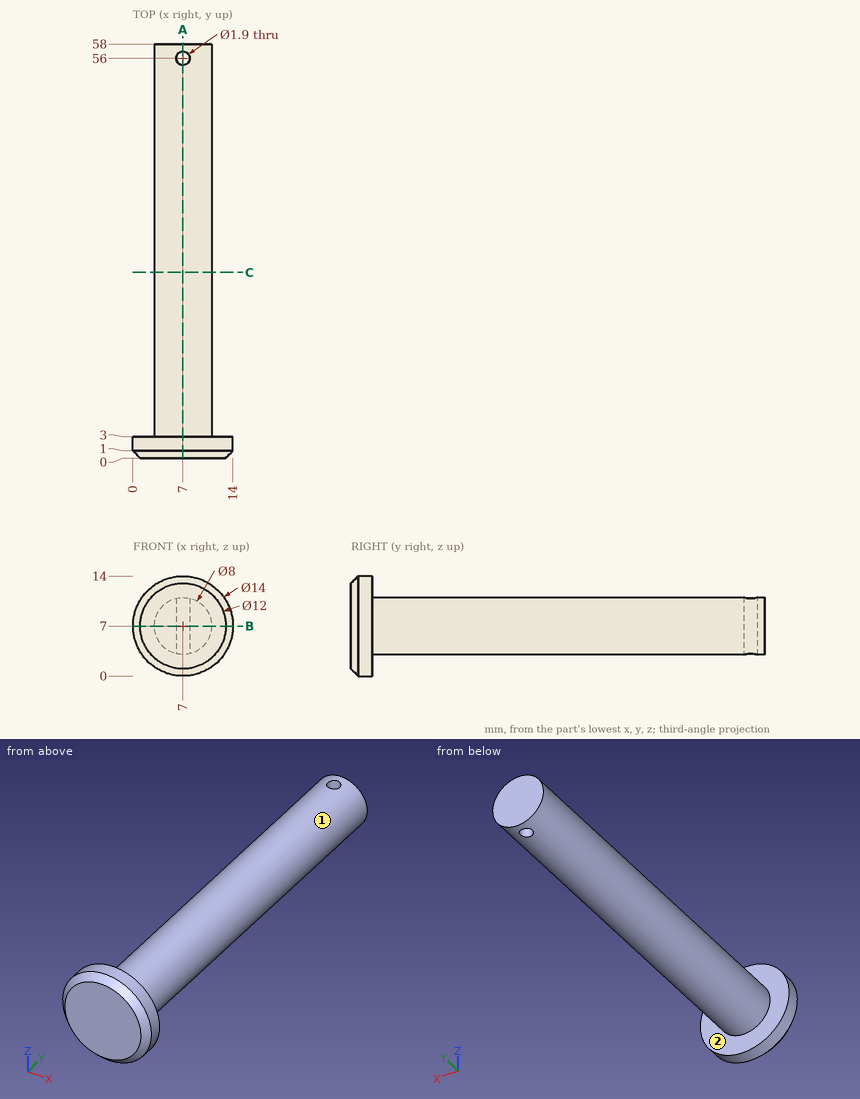
Answer from the drawing. Dimensions are ordinates in mm from the lowest x, y and z of the part. Coordinates: 2 decimals unless noted, no trailing zeros. Order: outer loops, then holes, each group sorted by start corner. A loop starts at its lowest first (then second) coordinate and runs counter-clockwise, first axis right, second up. Notation, with made-up numbers: M 41,4 L 70,4 A30 ccw 70,28 Z; hole C 27,69.5 d11. An arc over 180 degrees is marked long. Put each result on its own line as item: value. Start each with the question number.
Item 1: The mould has two halves that part along Z. Classify the marked faces 1 and 2: +Z half, -Z half, draft (parallel to the pull), parting line (faces both ways), or undercut.
Item 2: Section C-C, the plane y = 26 is taken. Determine the outline of the cut face in (x, z), plus the area to 3 significant figures.
Item 3: Given pin 1 Ø5 at (x, y) = (8, 21.5) entering from -Z; pin 2 Ø1.5 at (y, z) = (9, 7.5) entering from +X; pin 3 Ø6 at (x, y) = (8.5, 18) entering from +Z, each flat-ended and moving along its own axis, determine where each tip first touches the part or whether it passes through.
Item 4: Consider probe 1 along Y at (x, z) = (7, 5.75); probe 2 along Y at (x, z) = (11, 8.75); probe 3 along Z at (x, y) = (7.25, 49). Determine where each line is inside the solid, lowest interval first. Write a range as [from, to].
Item 5: Section A-A, the plane x = 7 is taken. Determine the outline of the cut face in (y, z).
Item 6: Section B-B, the plane z = 7 is taken. Determine the outline of the cut face in (x, y).
Computed:
1. face 1: parting line
1. face 2: draft
2. outline: C 7,7 d8
2. area: 50.3 mm2
3. pin 1: stops at z = 3
3. pin 2: stops at x = 11
3. pin 3: stops at z = 11
4. probe 1: y = [0, 55.05], [56.95, 58]
4. probe 2: y = [0, 3]
4. probe 3: z = [3.01, 10.99]
5. outline: M 0,1 L 1,0 L 3,0 L 3,3 L 55.05,3 L 55.05,11 L 3,11 L 3,14 L 1,14 L 0,13 Z; M 56.95,3 L 58,3 L 58,11 L 56.95,11 Z
6. outline: M 0,1 L 1,0 L 13,0 L 14,1 L 14,3 L 11,3 L 11,58 L 3,58 L 3,3 L 0,3 Z; hole C 7,56 d1.9
